Design review of the part built by this model. Coordinates are the model's own, in mm. A direction names the side the tool comes from. Round coordinates to 2 decimals unless told otherwise and drop trailing zeros. Loops run counter-clockwise (first coordinate to the right, second up) from the corner with the lowest first, then second, coordinate; pieces in that order, holes last. Notation, with made-up numbers: (-10.75, 85.25) -> (20.25, 85.25) arc R22 ccw to (20.25, 92.25) -> close; hole circle Ø6 at (57.25, -19). An arc over 180 degrees is marked (long way). Answer as CSV lines item,"result". Start each with the question number.
(1) Take a section at A-A, the plane z = 60. Write out the cut boundary in (x, y), and give its area (3 significant figures).
(2) Take a section at B-B, the plane x = 61. Write out the cut boundary in (y, z), and give its area (3 significant figures).
(3) Take a section at D-D, the plane y = 44. Write out the cut boundary in (x, z), and give its area (3 significant figures).
(4) For P1, Ø12, axis at y = -41.5, z = -19, coming from the +X side; P2, Ø6, axis at y = 44.5, z = -52.5, coming from the -X side; P3, Ø10, axis at x = -73, z = 23.5, coming from the -Y side, all flat-tipped, find the tip position at first contact; note any pin that passes through.
(5) Take a section at C-C, the plane y = 0. Write out the cut boundary in (x, z).
(6) Machinability: for faces 1 (the face through (-14.985, 0.66, 88.43)), 2 (the face through (-97.976, -2.155, -8.704)), 3 (the face through (24, 98, -9)), which of the approach directions +Z, -Z, +X, -X, +Y, -Y give a long, thin tool a straight path to every point of the face, cutting with its end or side? Answer none if there is none.
(7) To check wall thickness, follow line 1 (Z direction, x = -15, y = 9.5); line 2 (Z direction, x = 67.5, y = 79); line 3 (Y direction, x = 41, z = 8). State the ranges of each line that lie inside material, in increasing order. Write a range as from..to.
(8) Draft analysis for pull direction Z (two halves, no side actions). For faces 4 (the face through (23, -1, -98.5)), 5 (the face through (36, -100, -1)), 6 (the face through (23, 1, 83.5)), 7 (the face through (25, -98, -9)), state which applies: +Z half, -Z half, draft (parallel to the pull), parting line (faces both ways), or undercut.
from build123d import *

# Parameters (mm, degrees)
F4_DEPTH  = 5
F6_DEPTH  = 5
F8_DEPTH  = 172
F9_R      = 15
F10_DEPTH = 10


with BuildPart() as f2:
    # F0 (on Front) → F2 (revolve)
    with BuildSketch(Plane.XZ):
        Polygon((10, 78.5), (0, 78.5), (0, -93.5), (10, -93.5), (10, -78.5), (50, -78.5), (50, 63.5), (10, 63.5), align=None)
    revolve(axis=Axis((0, 0, -2.2203251719), (0, 0, -1)))

    # F3 (on face) → F4 (join)
    with BuildSketch(Plane.XY.offset(78.5)):
        with BuildLine():
            Line((150, 100), (0, 100))
            ThreePointArc((0, 100), (-100, 0), (0, -100))
            Line((0, -100), (150, -100))
            Line((150, -100), (150, 100))
        make_face()
    extrude(amount=F4_DEPTH)

    # F5 (on face) → F6 (join)
    with BuildSketch(Plane(origin=(0, 0, -93.5), x_dir=(1, 0, 0), z_dir=(0, 0, -1))):
        with BuildLine():
            ThreePointArc((0, 100), (-100, 0), (0, -100))
            Line((0, -100), (150, -100))
            Line((150, -100), (150, 100))
            Line((150, 100), (0, 100))
        make_face()
    extrude(amount=F6_DEPTH)

    # F7 (on face) → F8 (join, through all)
    with BuildSketch(Plane.XY.offset(-93.5)):
        with BuildLine():
            Line((49, 100), (0, 100))
            ThreePointArc((0, 100), (-100, 0), (0, -100))
            Line((0, -100), (49, -100))
            Line((49, -100), (49, -98))
            Line((49, -98), (0, -98))
            ThreePointArc((0, -98), (-98, 0), (0, 98))
            Line((0, 98), (49, 98))
            Line((49, 98), (49, 100))
        make_face()
    extrude(amount=F8_DEPTH)

    # F9 (on face) → F10 (join)
    with BuildSketch(Plane.XY.offset(83.5)):
        Circle(F9_R)
    extrude(amount=F10_DEPTH)


solid = f2.part
The answers:
1,outline,"circle Ø100 at (0, 0); (0, -100) -> (49, -100) -> (49, -98) -> (0, -98) arc R98 cw to (0, 98) -> (49, 98) -> (49, 100) -> (0, 100) arc R100 ccw to start"
1,area,"8,670 mm²"
2,outline,"(-100, -98.5) -> (100, -98.5) -> (100, -93.5) -> (-100, -93.5) -> close; (-100, 78.5) -> (100, 78.5) -> (100, 83.5) -> (-100, 83.5) -> close"
2,area,"2,000 mm²"
3,outline,"(-89.8, -98.5) -> (150, -98.5) -> (150, -93.5) -> (-87.57, -93.5) -> (-87.57, 78.5) -> (150, 78.5) -> (150, 83.5) -> (-89.8, 83.5) -> close; (-23.75, -78.5) -> (23.75, -78.5) -> (23.75, 63.5) -> (-23.75, 63.5) -> close"
3,area,"9,530 mm²"
4,P1,"x = 35.21"
4,P2,"x = -90.98"
4,P3,"y = -73.32"
5,outline,"(-100, -98.5) -> (150, -98.5) -> (150, -93.5) -> (10, -93.5) -> (10, -78.5) -> (50, -78.5) -> (50, 63.5) -> (10, 63.5) -> (10, 78.5) -> (150, 78.5) -> (150, 83.5) -> (15, 83.5) -> (15, 93.5) -> (-15, 93.5) -> (-15, 83.5) -> (-100, 83.5) -> close; hole (-98, -93.5) -> (-10, -93.5) -> (-10, -78.5) -> (-50, -78.5) -> (-50, 63.5) -> (-10, 63.5) -> (-10, 78.5) -> (-98, 78.5) -> close"
6,face 1,"+Z"
6,face 2,"none"
6,face 3,"+X"
7,line 1,"-98.5..-93.5, -78.5..63.5, 78.5..83.5"
7,line 2,"-98.5..-93.5, 78.5..83.5"
7,line 3,"-100..-98, -28.62..28.62, 98..100"
8,face 4,"-Z half"
8,face 5,"draft"
8,face 6,"+Z half"
8,face 7,"undercut"
